The listing builds one solid part. Answer for the finished solid, in the listing's coordinates (mm). A direction names the side the tool comes from. Give positions to 0.01 mm unless a question says otherwise; leave off trailing zeros. Write each loop counter-clockwise with the first axis right and the second up, starting at its lowest first coordinate (ties: lowest second). Pieces come first, ordered by that corner, then holes.
```python
from build123d import *

# Parameters (mm, degrees)
SKETCH1_R           = 28
BOSS_EXTRUDE1_DEPTH = 8
SKETCH2_R           = 15
CUT_EXTRUDE1_DEPTH  = 43.708313008
CHAMFER1_SIZE       = 1
CUT_EXTRUDE2_DEPTH  = 4


with BuildPart() as part:
    # Sketch1 → Boss-Extrude1 (new, symmetric)
    with BuildSketch(Plane(origin=(0, 0, 0), x_dir=(0, 0, -1), z_dir=(1, 0, 0))):
        Circle(SKETCH1_R)
    extrude(amount=BOSS_EXTRUDE1_DEPTH, both=True)

    # Sketch2 → Cut-Extrude1 (cut, through all)
    with BuildSketch(Plane(origin=(8, 0, 0), x_dir=(0, 0, -1), z_dir=(1, 0, 0))):
        with Locations((0, 38)):
            Circle(SKETCH2_R)
    extrude(amount=-CUT_EXTRUDE1_DEPTH, mode=Mode.SUBTRACT)

    # Chamfer1
    chamfer1_edges = [part.edges().sort_by_distance(p)[0] for p in [
        (-8, -28, 0),
        (8, -28, 0),
        (8, 23, 0),
        (-8, 23, 0),
    ]]
    chamfer(chamfer1_edges, length=CHAMFER1_SIZE)

    # Sketch3 → Cut-Extrude2 (cut)
    with BuildSketch(Plane(origin=(8, 0, 0), x_dir=(0, 0, -1), z_dir=(1, 0, 0))):
        with BuildLine():
            ThreePointArc((-9.89010775, 22.960526316), (0, -25), (9.89010775, 22.960526316))
            ThreePointArc((9.89010775, 22.960526316), (0, 20), (-9.89010775, 22.960526316))
        make_face()
    cut_extrude2 = extrude(amount=-CUT_EXTRUDE2_DEPTH, mode=Mode.SUBTRACT)

    # Mirror1: Cut-Extrude2 across plane
    add(cut_extrude2.mirror(Plane(origin=(0, 0, 0), x_dir=(0, 0, 1), z_dir=(1, 0, 0))), mode=Mode.SUBTRACT)


solid = part.part
```
Item 1: Each of these flat-tipped pins is pushed along its axis until it touches: P1, Ø4, axis at y = -1.5, z = -19, coming from the +X side; P2, Ø5, axis at x = 0.5, z = -1.5, coming from the -Y side; P3, Ø10, axis at y = -1.5, z = -3, coming from the -X side. Where does it stop, or does it pass through?
Conclusion:
P1: stops at x = 4
P2: stops at y = -28
P3: stops at x = -4
Item 2: A cutting plane is placed at B-B, the plane z = 0. Give the vertices of the cut face in (x, y), plus the area to 3 significant figures.
Conclusion:
outline: (-8, -27) - (-7, -28) - (7, -28) - (8, -27) - (8, -25) - (4, -25) - (4, 20) - (8, 20) - (8, 22) - (7, 23) - (-7, 23) - (-8, 22) - (-8, 20) - (-4, 20) - (-4, -25) - (-8, -25) - close
area: 454 mm2
Item 3: A cutting plane is placed at A-A, the plane y = 0. Give the vertices of the cut face in (x, z), plus the area to 3 significant figures.
Conclusion:
outline: (-8, -27) - (-7, -28) - (7, -28) - (8, -27) - (8, -25) - (4, -25) - (4, 25) - (8, 25) - (8, 27) - (7, 28) - (-7, 28) - (-8, 27) - (-8, 25) - (-4, 25) - (-4, -25) - (-8, -25) - close
area: 494 mm2
Item 4: Consider probe 1 along Z at (x, y) = (6.5, 0); probe 2 along X at (y, z) = (-19, 13.5); probe 3 along Z at (x, y) = (5.75, 6). Determine where each line is inside the solid, lowest interval first.
Conclusion:
probe 1: z = -28 to -25, 25 to 28
probe 2: x = -4 to 4
probe 3: z = -27.35 to -24.27, 24.27 to 27.35
Item 5: Which of the six approach directions +Z, -Z, +X, -X, +Y, -Y give full straight-line access (tool end or side, diameter ignored) to faces 4 (the face through (-6.03, -24.98, 0.96)), 5 (the face through (7.2, 22.8, 0.1)), 6 (the face through (6, 20, 0))?
Conclusion:
face 4: -X
face 5: +X, +Y
face 6: +X
Item 6: A cutting plane is placed at C-C, the plane x = 5.5. Give the vertices of the cut face in (y, z), plus the area to 3 significant figures.
Conclusion:
outline: (26.36, -9.46) arc R15 cw to (26.36, 9.46) arc R28 ccw (long way) to start; hole (22.96, -9.89) arc R18 cw to (22.96, 9.89) arc R25 ccw (long way) to start
area: 502 mm2
Item 7: Determine the mould class of faces 1 (the face through (0.1, -27.98, 1.1)), 2 (the face through (-6, 20, 0)), 3 (the face through (0, 23, 0)) for opening direction Y: pulls with the +Y half, pulls with the -Y half, needs draft (parallel to the pull), parting line crosses it, or undercut.
Conclusion:
face 1: parting line crosses it
face 2: undercut
face 3: pulls with the +Y half
